from build123d import *

# Parameters (mm, degrees)
SKETCH1_R           = 30
SKETCH1_R_2         = 5
SKETCH1_R_3         = 0.7
BOSS_EXTRUDE1_DEPTH = 3
BOSS_EXTRUDE2_DEPTH = 3
CIRPATTERN2_COUNT   = 24


with BuildPart() as part:
    # Sketch1 → Boss-Extrude1 (new body)
    with BuildSketch(Plane.XY):
        Circle(SKETCH1_R)
        Circle(SKETCH1_R_2, mode=Mode.SUBTRACT)
        with Locations((-3.5, 7.25)):
            Circle(SKETCH1_R_3, mode=Mode.SUBTRACT)
        with Locations((0, 7.25)):
            Circle(SKETCH1_R_3, mode=Mode.SUBTRACT)
        with Locations((3.5, 7.25)):
            Circle(SKETCH1_R_3, mode=Mode.SUBTRACT)
        with Locations((7.25, 3.5)):
            Circle(SKETCH1_R_3, mode=Mode.SUBTRACT)
        with Locations((7.25, 0)):
            Circle(SKETCH1_R_3, mode=Mode.SUBTRACT)
        with Locations((7.25, -3.5)):
            Circle(SKETCH1_R_3, mode=Mode.SUBTRACT)
        with Locations((3.5, -7.25)):
            Circle(SKETCH1_R_3, mode=Mode.SUBTRACT)
        with Locations((0, -7.25)):
            Circle(SKETCH1_R_3, mode=Mode.SUBTRACT)
        with Locations((-3.5, -7.25)):
            Circle(SKETCH1_R_3, mode=Mode.SUBTRACT)
        with Locations((-7.25, -3.5)):
            Circle(SKETCH1_R_3, mode=Mode.SUBTRACT)
        with Locations((-7.25, 0)):
            Circle(SKETCH1_R_3, mode=Mode.SUBTRACT)
        with Locations((-7.25, 3.5)):
            Circle(SKETCH1_R_3, mode=Mode.SUBTRACT)
    extrude(amount=BOSS_EXTRUDE1_DEPTH)

    # Sketch2 → Boss-Extrude2 (add)
    with BuildSketch(Plane.XY.offset(3)):
        with BuildLine():
            Line((29.948176492, 1.762590363), (31.948176492, 1.762590363))
            ThreePointArc((31.948176492, 1.762590363), (32.655283273, 1.469697144), (32.948176492, 0.762590363))
            Line((32.948176492, 0.762590363), (32.948176492, -0.762590363))
            ThreePointArc((32.948176492, -0.762590363), (32.655283273, -1.469697144), (31.948176492, -1.762590363))
            Line((31.948176492, -1.762590363), (29.948176492, -1.762590363))
            Line((29.948176492, -1.762590363), (29.948176492, 1.762590363))
        make_face()
    boss_extrude2 = extrude(amount=-BOSS_EXTRUDE2_DEPTH)

    # CirPattern2: Boss-Extrude2 ×24 about axis
    cirpattern2_axis = Axis((0, 0, 0), (0, 0, 1))
    for i in range(1, CIRPATTERN2_COUNT):
        add(boss_extrude2.rotate(cirpattern2_axis, i * 360 / CIRPATTERN2_COUNT))


solid = part.part
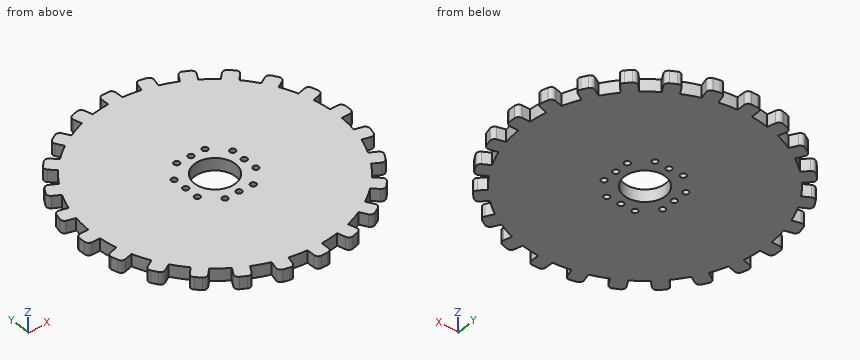
The listing builds one solid part. Answer for the finished solid, in the listing's coordinates (mm). Round coordinates to 2 decimals unless told otherwise and drop trailing zeros. Write each question's results on one line, items separated by ' | '. Start each with the question number.
(1) Find the intervals of material crossed by line 1 (Y direction, x = 0, z = 2.25); line 2 (X direction, y = 27, z = 1.3); line 3 (X direction, y = 17.5, z = 1.6), in increasing order.
(2) Each of these flat-tipped pins is pushed along its axis until it touches: P1, Ø0.6, axis at y = 30.5, z = 1.5, coming from the +X side; P2, Ø0.6, axis at y = -31.5, z = 1.5, coming from the +X side; P3, Ø1, axis at y = -26.5, z = 1.5, coming from the +X side. Where does it stop, or does it pass through?
(3) The part is cut by section A-A, the plane z = 1.6. Give the number of separate pieces and of enclosed holes in the cut face, and give its area (3 significant figures).
Worked answers:
1) line 1: y = -32.95 to -7.95, -6.55 to -5, 5 to 6.55, 7.95 to 32.95 | line 2: x = -17.59 to -13.55, -13.08 to 13.08, 13.55 to 17.59 | line 3: x = -27.79 to -26.79, -24.37 to 24.37, 26.79 to 27.79
2) P1: stops at x = 10.01 | P2: stops at x = 9.85 | P3: stops at x = 17.59
3) separate pieces: 1 | enclosed holes: 13 | area: 2,970 mm²
